Verification items for the finished model (mm, model axes). Face numbers are marked on the shaded views. A direction names the side the tool comes from. Coordinates: 2 decimals unless noted, no trailing zeros. Order: outer loops, then holes, each group sorted by start corner. A loop starts at its lowest first (then second) coordinate and runs counter-clockwise, first axis right, second up. Notation, with made-up numbers: (11.5, 19) -> (45.5, 19) arc R12 cw to (45.5, 34) -> close; hole circle Ø2 at (75.25, 81.25). An arc over 180 degrees is marked (long way). Use CSV: the item, a comma, the result in double quotes. Start each with the question number.
1) Scan lines: line 1 along X through (y, z) = (-80, 8); line 2 along X through (y, z) = (-117, 9); line 3 along Z through (x, y) = (10, -114). Record each from-to range of solid material in increasing order.
2) Go/stop test with flat-tipped pins: pin 1 (3 mm diameter, centred on y = -114, z = 5, fed in from -X); pin 2 (3 mm diameter, centred on y = -110.5, z = 4.5, fed in from +X); pin 3 (3 mm diameter, centred on x = -11.5, z = 7, fed in from -Y). Record where each tip stops, or that it passes through.
3) Release check for a two-part mould opening along Y. For the marked faces 4, 5 and 6 record: released by +Y, released by -Y, zero draft, split by the parting line, or undercut.
4) Tool access check on the marked faces 1, 2 and 3. Record the directions out of +Z, -Z, +X, -X, +Y, -Y that give a thin tool (end or side, any length) a straight path to the whole face; none if there is none.
5) Sectioned sample at B-B on y = -109.5. Record the boundary of the cut face in (x, z), then the cut area to 3 significant figures.
6) Sectioned sample at C-C on x = 4.5. Record the boundary of the cut face in (y, z).
7) Sectioned sample at D-D on x = 15. Record the boundary of the cut face in (y, z), then the cut area to 3 significant figures.
8) Sectioned sample at A-A on y = -114. Record the boundary of the cut face in (x, z), then the cut area to 3 significant figures.
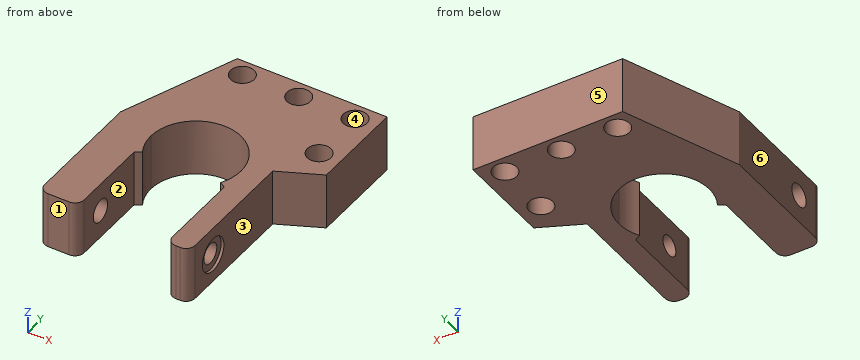
from build123d import *

# Parameters (mm, degrees)
CYLINDER011012_R               = 1.8
CYLINDER011012_DEPTH           = 20
CYLINDER011013_R               = 3
CYLINDER011013_DEPTH           = 20
BOX010_W                       = 20
BOX010_H                       = 10
BOX010_DEPTH                   = 20
CYLINDER011029_R               = 2.1
CYLINDER011029_DEPTH           = 20
ARRAY017_X_COUNT               = 4
ARRAY017_X_PITCH               = 10
ARRAY017_Y_COUNT               = 2
ARRAY017_Y_PITCH               = 10
CYLINDER011011_R               = 2
CYLINDER011011_DEPTH           = 20
CYLINDER011014_R               = 8
CYLINDER011014_DEPTH           = 10
CYLINDER011015_W               = 11
CYLINDER011015_H               = 10
CYLINDER011015_ANGLE           = 240
CYLINDER011015_PLACEMENT_ANGLE = 150
PAD_DEPTH                      = 10


with BuildPart() as bolt_hole001:
    # Cylinder011012 → Cylinder011012 (new body)
    with BuildSketch(Plane(origin=(-1, 14, 5), x_dir=(0, 0, -1), z_dir=(1, 0, 0))):
        Circle(CYLINDER011012_R)
    extrude(amount=CYLINDER011012_DEPTH)


with BuildPart() as bolt_head_hole:
    # Cylinder011013 → Cylinder011013 (new body)
    with BuildSketch(Plane(origin=(11.5, 14, 5), x_dir=(0, 0, -1), z_dir=(1, 0, 0))):
        Circle(CYLINDER011013_R)
    extrude(amount=CYLINDER011013_DEPTH)


with BuildPart() as cube:
    # Box010 → Box010 (new body)
    with BuildSketch(Plane(origin=(-9, -14, 0), x_dir=(1, 0, 0), z_dir=(0, 0, 1))):
        with Locations((10, 5)):
            Rectangle(BOX010_W, BOX010_H)
    extrude(amount=BOX010_DEPTH)


with BuildPart() as general_insert_hole_array_cut:
    # Cylinder011029 → Cylinder011029 (new body)
    with BuildSketch(Plane.XY):
        Circle(CYLINDER011029_R)
    extrude(amount=CYLINDER011029_DEPTH)

    # Array017 X: general insert hole array cut ×4


with BuildPart() as general_insert_hole_array_cut_1:
    add(general_insert_hole_array_cut.part)
    with Locations(*[(i * ARRAY017_X_PITCH, 0, 0) for i in range(1, ARRAY017_X_COUNT)]):
        add(general_insert_hole_array_cut.part)

    # Array017 Y: general insert hole array cut ×2


with BuildPart() as general_insert_hole_array_cut_2:
    add(general_insert_hole_array_cut_1.part)
    with Locations(*[(0, i * ARRAY017_Y_PITCH, 0) for i in range(1, ARRAY017_Y_COUNT)]):
        add(general_insert_hole_array_cut_1.part)


with BuildPart() as general_insert_hole_array_cut_3:
    # Array017 placement: moved
    add(general_insert_hole_array_cut_2.part.moved(Location((-4.5, -20, 0))))

    # Cut023015009020: cut Cube
    add(cube.part, mode=Mode.SUBTRACT)


with BuildPart() as shaft_attachment_hole_fusion:
    # Cylinder011011 → Cylinder011011 (new body)
    with BuildSketch(Plane(origin=(-22, 14, 5), x_dir=(0, 0, -1), z_dir=(1, 0, 0))):
        Circle(CYLINDER011011_R)
    extrude(amount=CYLINDER011011_DEPTH)

    # Fusion004: union bolt hole001, bolt head hole, general insert hole array cut
    add(bolt_hole001.part)
    add(bolt_head_hole.part)
    add(general_insert_hole_array_cut_3.part)


with BuildPart() as cylinder:
    # Cylinder011014 → Cylinder011014 (new body)
    with BuildSketch(Plane.XY):
        Circle(CYLINDER011014_R)
    extrude(amount=CYLINDER011014_DEPTH)


with BuildPart() as cut023015009010:
    # Cylinder011015 → Cylinder011015 (revolve)
    with BuildSketch(Plane.XZ):
        with Locations((5.5, 5)):
            Rectangle(CYLINDER011015_W, CYLINDER011015_H)
    revolve(axis=Axis((0, 0, 0), (0, 0, 1)), revolution_arc=CYLINDER011015_ANGLE)


with BuildPart() as cut023015009010_1:
    # Cylinder011015 placement: moved
    add(cut023015009010.part.rotate(Axis((0, 0, 0), (0, 0, 1)), CYLINDER011015_PLACEMENT_ANGLE))

    # Cut023015009010: cut Cylinder
    add(cylinder.part, mode=Mode.SUBTRACT)


with BuildPart() as shaft_attachment_cut:
    # Sketch002 → Pad (new body)
    with BuildSketch(Plane.XY):
        with BuildLine():
            Line((12, -2.57721), (12, 19.017869))
            ThreePointArc((12, 19.017869), (11.523224, 20.168908), (10.372186, 20.645684))
            Line((10.372186, 20.645684), (9.627814, 20.645684))
            ThreePointArc((9.627814, 20.645684), (8.476776, 20.168908), (8, 19.017869))
            Line((8, 19.017869), (8, 0))
            ThreePointArc((-8, 0), (0, -8), (8, 0))
            Line((-8, 0), (-8, 18.544726))
            ThreePointArc((-8, 18.544726), (-8.476776, 19.695765), (-9.627814, 20.17254))
            Line((-9.627814, 20.17254), (-13.372186, 20.17254))
            ThreePointArc((-13.372186, 20.17254), (-14.523224, 19.695765), (-15, 18.544726))
            Line((-15, 18.544726), (-15, -2.57721))
            Line((-15, -2.57721), (-7.274933, -22.958025))
            Line((-7.274933, -22.958025), (19.286886, -22.958025))
            Line((19.286886, -22.958025), (19.286886, -6.082279))
            Line((19.286886, -6.082279), (12, -2.57721))
        make_face()
    extrude(amount=PAD_DEPTH)

    # Fusion005: union Cut023015009010
    add(cut023015009010_1.part)

    # Cut023015009009: cut shaft attachment hole fusion
    add(shaft_attachment_hole_fusion.part, mode=Mode.SUBTRACT)


with BuildPart() as part_mirroring001:
    # Part__Mirroring001: instance of shaft attachment  cut
    add(shaft_attachment_cut.part.mirror(Plane(origin=(0, -50, 0), x_dir=(1, 0, 0), z_dir=(0, 1, 0))))


solid = part_mirroring001.part
Answers follow:
1,line 1,"x = -8.4 to -6.6, -2.4 to 3.4, 7.6 to 13.4, 17.6 to 19.29"
1,line 2,"x = -15 to -8, 8 to 12"
1,line 3,"z = 0 to 3.2, 6.8 to 10"
2,pin 1,"passes through"
2,pin 2,"stops at x = 12"
2,pin 3,"stops at y = -120.17"
3,face 4,"undercut"
3,face 5,"released by +Y"
3,face 6,"zero draft"
4,face 1,"+Z, -Z, -X, -Y"
4,face 2,"+Z, -Z, -Y"
4,face 3,"+Z, -Z, +X, -Y"
5,outline,"(-15, 0) -> (-8, 0) -> (-8, 10) -> (-15, 10) -> close; (8, 0) -> (12, 0) -> (12, 10) -> (8, 10) -> close"
5,area,"110 mm²"
6,outline,"(-93.39, 0) -> (-81.85, 0) -> (-81.85, 10) -> (-93.39, 10) -> close; (-78.15, 0) -> (-77.04, 0) -> (-77.04, 10) -> (-78.15, 10) -> close"
7,outline,"(-95.98, 0) -> (-92.04, 0) -> (-92.04, 10) -> (-95.98, 10) -> close; (-87.96, 0) -> (-82.04, 0) -> (-82.04, 10) -> (-87.96, 10) -> close; (-77.96, 0) -> (-77.04, 0) -> (-77.04, 10) -> (-77.96, 10) -> close"
7,area,"108 mm²"
8,outline,"(-15, 0) -> (-8, 0) -> (-8, 3) -> (-15, 3) -> close; (-15, 7) -> (-8, 7) -> (-8, 10) -> (-15, 10) -> close; (8, 0) -> (12, 0) -> (12, 2) -> (11.5, 2) -> (11.5, 3.2) -> (8, 3.2) -> close; (8, 6.8) -> (11.5, 6.8) -> (11.5, 8) -> (12, 8) -> (12, 10) -> (8, 10) -> close"
8,area,"66.4 mm²"
